Check sheet for the drawn part. Datum: minimum x, y, z corner. Units: mm. Coordinates: 2 decimals unless noted, no trailing zeros. Loops run counter-clockwise (first coordinate to the right, second up) from the corner with the lowest first, then second, coordinate; pieces in that order, holes last.
Q1. Sectioned sample at B-B (x = 267). Enter the section's corners in (y, z), then the cut area to 3 significant figures.
Q2. Material ranges on probe 1 along X at (y, z) = (4.25, 155.5); probe 2 along Z at (x, y) = (14, 2.5); probe 3 along X at (y, z) = (5.75, 69), recorded low to high.
Q3. Go/stop test with a flat-tipped pin: P1, Ø5, axis at x = 280, z = 10, coming from the +Y side. Record where the tip stops, or that it passes through.
Q4. Sectioned sample at A-A (y = 8.25). Count the separate pieces of the cut face and the enclosed holes in it, then the cut area to 3 significant figures.
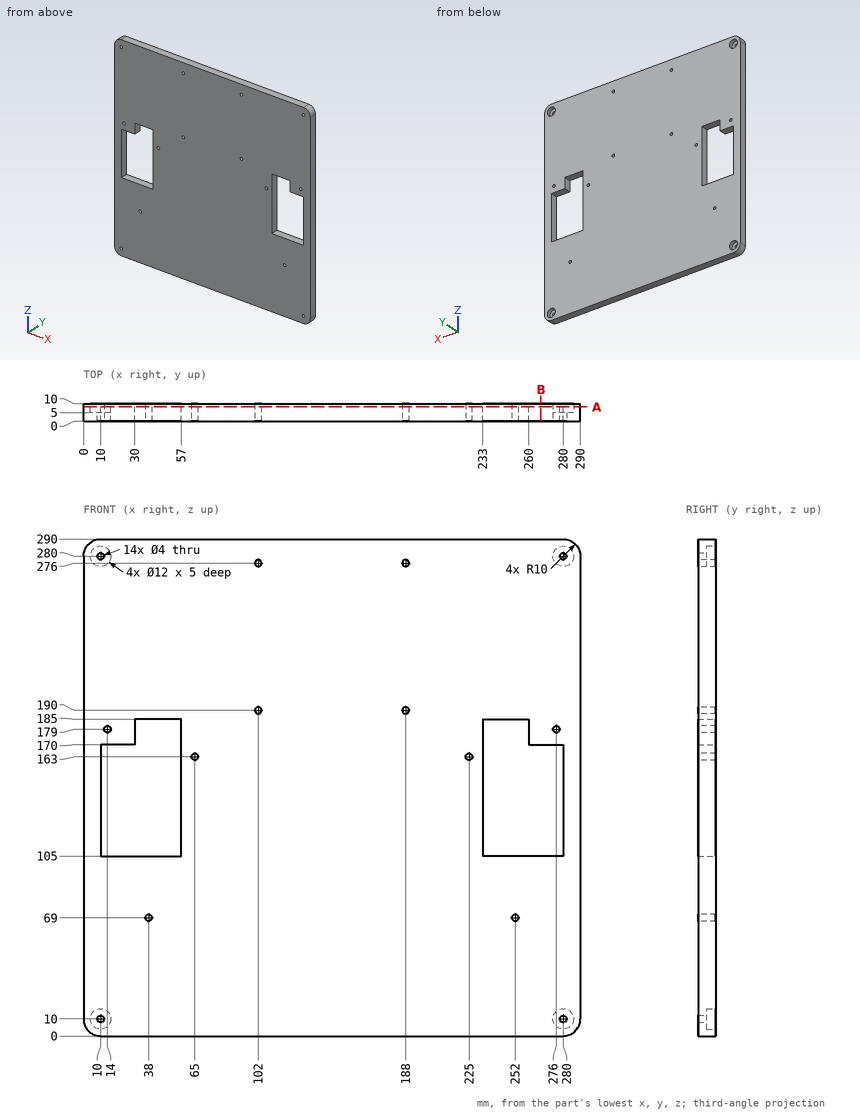
Geometry check:
1. outline: (0, 0) - (10, 0) - (10, 105) - (0, 105) - close; (0, 170) - (10, 170) - (10, 290) - (0, 290) - close
1. area: 2,250 mm2
2. probe 1: x = 0 to 10, 57 to 233, 280 to 290
2. probe 2: z = 0 to 105, 170 to 177, 181 to 290
2. probe 3: x = 0 to 36, 40 to 250, 254 to 290
3. P1: stops at y = 5
4. separate pieces: 1
4. enclosed holes: 16
4. area: 76,500 mm2
